Geometry: see drawing. Coordinates: mm, zero at the bounding-box minimum. A direction names the side the tool comes from. Coordinates: 2 decimals unless noted, no trailing zeros. Write each loop counter-clockwise with the first axis right and the second up, starting at its lowest first coordinate (ties: lowest second). Pieces come first, ordered by that corner, then holes.
1) Line query: L1, parallel to X at y = 8, z = 2; L2, parallel to Y at x = 26, z = 4.25; L3, parallel to Z at x = 22.5, y = 10.75. Output: solid intervals per line, ascending.
2) Pin query (flat end, axial travel): pin 1 Ø12 at (x, y) = (35, 15.5) entering from +Z. Return the tip coordinate at first contact, or that it passes through.
3) Section query C-C (z = 9.5). Output: boundary loops of the cut face in (x, y), then the cut area to 3 significant figures.
4) Section query B-B (y = 12.5). Output: boundary loops of the cut face in (x, z), then the cut area to 3 significant figures.
5) Draft query along X for the marked faces 3, 4, 5 and 6. Return one class per face: pulls with the +X half, pulls with the -X half, needs draft (parallel to the pull), parting line crosses it, or undercut.
6) Set-up query: the marked faces 1 and 2. Return all of +Z, -Z, +X, -X, +Y, -Y with unobstructed straight access to the full face (end or side cutting, diameter ignored); none if empty.
7) Section query A-A (z = 2.5). Output: boundary loops of the cut face in (x, y), then the cut area to 3 significant figures.
8) Section query D-D (x = 7). Output: boundary loops of the cut face in (y, z), then the cut area to 3 significant figures.
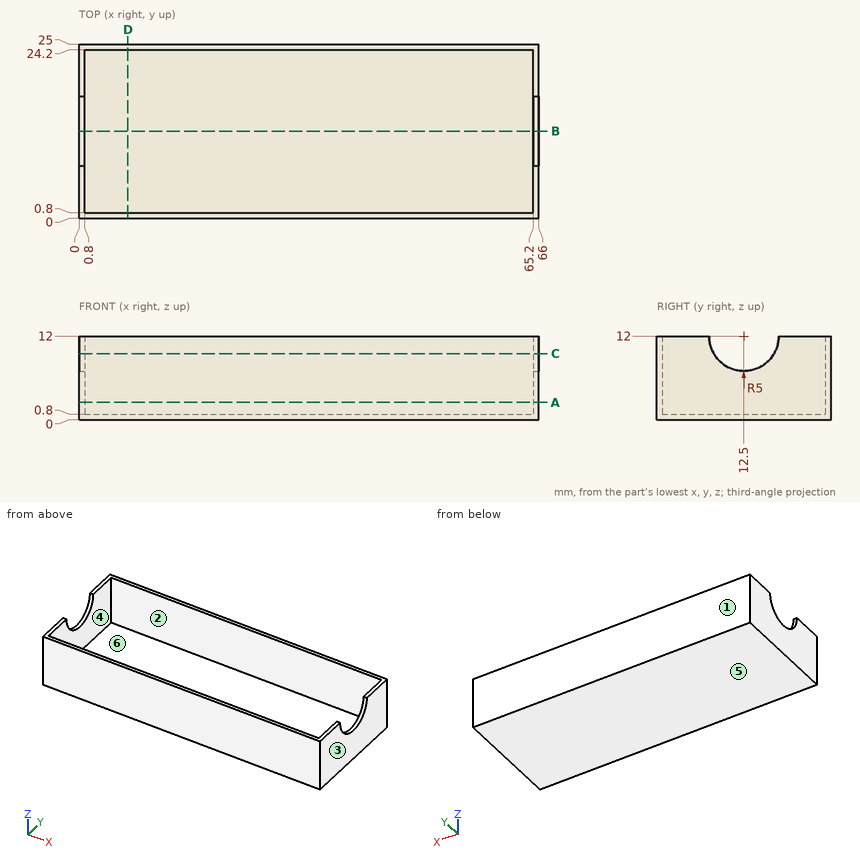
Answer:
1. L1: x = 0 to 0.8, 65.2 to 66
1. L2: y = 0 to 0.8, 24.2 to 25
1. L3: z = 0 to 0.8
2. pin 1: stops at z = 0.8
3. outline: (0, 0) - (66, 0) - (66, 8.17) - (65.2, 8.17) - (65.2, 0.8) - (0.8, 0.8) - (0.8, 8.17) - (0, 8.17) - close; (0, 16.83) - (0.8, 16.83) - (0.8, 24.2) - (65.2, 24.2) - (65.2, 16.83) - (66, 16.83) - (66, 25) - (0, 25) - close
3. area: 129 mm2
4. outline: (0, 0) - (66, 0) - (66, 7) - (65.2, 7) - (65.2, 0.8) - (0.8, 0.8) - (0.8, 7) - (0, 7) - close
4. area: 62.7 mm2
5. face 3: pulls with the +X half
5. face 4: undercut
5. face 5: needs draft
5. face 6: undercut
6. face 1: +Z, -Z, +X, -X, +Y
6. face 2: +Z
7. outline: (0, 0) - (66, 0) - (66, 25) - (0, 25) - close; hole (0.8, 0.8) - (65.2, 0.8) - (65.2, 24.2) - (0.8, 24.2) - close
7. area: 143 mm2
8. outline: (0, 0) - (25, 0) - (25, 12) - (24.2, 12) - (24.2, 0.8) - (0.8, 0.8) - (0.8, 12) - (0, 12) - close
8. area: 37.9 mm2
